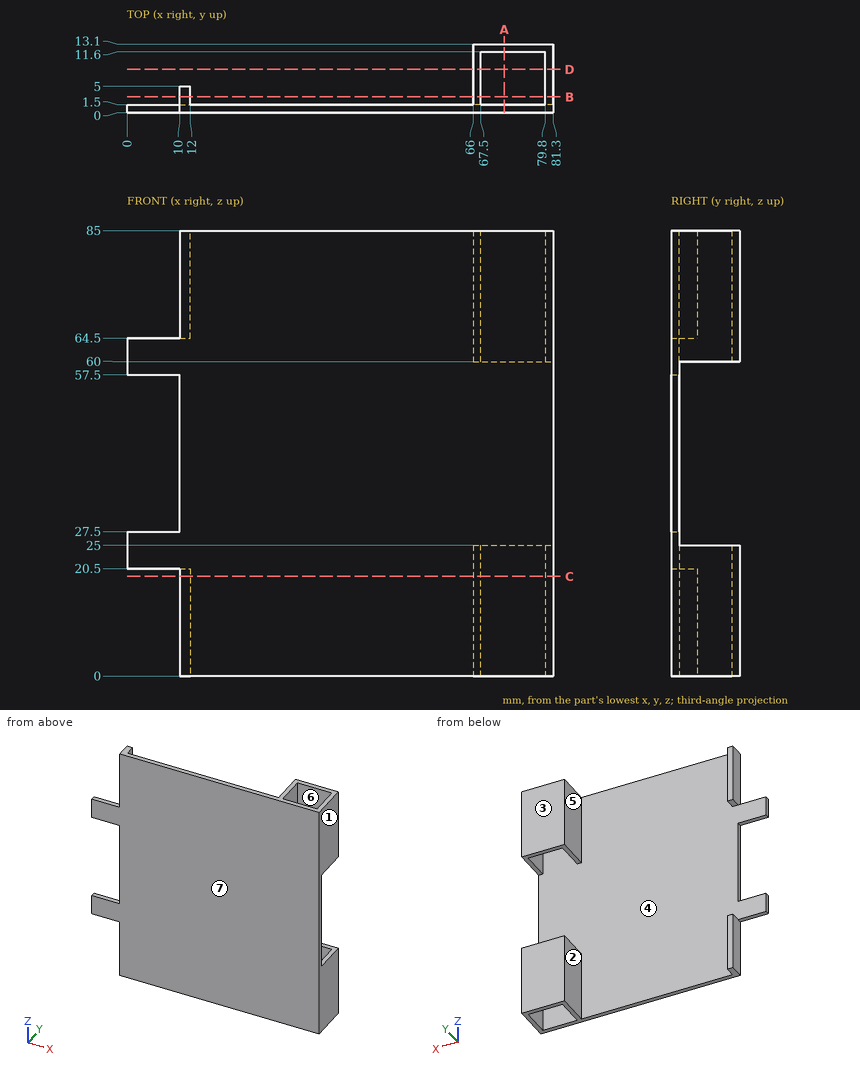
Could you check a few things on this drawing? It's one solid part, dimensions in mm from its lowest x, y, z. A direction names the side the tool comes from. Coordinates: 2 decimals unless noted, no trailing zeros. Write each loop counter-clockwise with the first axis right and the second up, starting at its lowest first coordinate (ties: lowest second). Pieces come first, ordered by that corner, then holes. Notation, with made-up numbers: M 75.25,21.25 L 83.25,21.25 A11 cw 83.25,32.25 Z; hole C -33,-27.5 d2. An arc over 180 degrees is marked long. Answer as CSV lines item,"result". Start each with the question number.
Q1. Suppose I cut it at B-B, the plane y = 3. List the corners of the cut face in (x, z) for me.
Q2. Suppose I cut it at C-C, the plane z = 19. List the corners of the cut face in (x, y) for me.
Q3. Suppose I cut it at D-D, the plane y = 8.25. List the corners of the cut face in (x, z) for me.
Q4. Will these pins go through, and if not, where does the flat tip stop? pin 1 Ø5 at (y, z) = (8.5, 18) entering from -X; pin 2 Ø4 at (y, z) = (3, 12.5) entering from -X; pin 3 Ø10 at (x, z) = (55.5, 38) entering from +Y.
Q5. I need wall thicknesses on probe 1 along X at (y, z) = (4, 80); probe 2 along X at (y, z) = (2.5, 21); probe 3 along Y at (x, z) = (31.5, 38). Which ranges of each line are inside material? Lowest first, please. Write a range as [from, to].
Q6. Suppose I cut it at A-A, the plane x = 72. List the corners of the cut face in (y, z) for me.
Q7. For the marked faces 5, 6 and 7, which set-ups out of +Z, -Z, +X, -X, +Y, -Y let a thin tool reach every point of the face, with its end or its side?
Q8. If we mould it in two halves opening along X, with no side actions, what happens to the marked faces 1, 2, 3 and 4? For each: pulls with the +X half, pulls with the -X half, needs draft (parallel to the pull), parting line crosses it, or undercut.
Entries:
1,outline,"M 10,0 L 12,0 L 12,20.5 L 10,20.5 Z; M 10,64.5 L 12,64.5 L 12,85 L 10,85 Z; M 66,0 L 67.5,0 L 67.5,25 L 66,25 Z; M 66,60 L 67.5,60 L 67.5,85 L 66,85 Z; M 79.8,0 L 81.3,0 L 81.3,25 L 79.8,25 Z; M 79.8,60 L 81.3,60 L 81.3,85 L 79.8,85 Z"
2,outline,"M 10,0 L 81.3,0 L 81.3,13.1 L 66,13.1 L 66,1.5 L 12,1.5 L 12,5 L 10,5 Z; hole M 67.5,1.5 L 79.8,1.5 L 79.8,11.6 L 67.5,11.6 Z"
3,outline,"M 66,0 L 67.5,0 L 67.5,25 L 66,25 Z; M 66,60 L 67.5,60 L 67.5,85 L 66,85 Z; M 79.8,0 L 81.3,0 L 81.3,25 L 79.8,25 Z; M 79.8,60 L 81.3,60 L 81.3,85 L 79.8,85 Z"
4,pin 1,"stops at x = 66"
4,pin 2,"stops at x = 10"
4,pin 3,"stops at y = 1.5"
5,probe 1,"x = [10, 12], [66, 67.5], [79.8, 81.3]"
5,probe 2,"x = [66, 67.5], [79.8, 81.3]"
5,probe 3,"y = [0, 1.5]"
6,outline,"M 0,0 L 1.5,0 L 1.5,85 L 0,85 Z; M 11.6,0 L 13.1,0 L 13.1,25 L 11.6,25 Z; M 11.6,60 L 13.1,60 L 13.1,85 L 11.6,85 Z"
7,face 5,"+Z, -Z, +Y"
7,face 6,"+Z, -Z"
7,face 7,"+Z, -Z, +X, -X, -Y"
8,face 1,"pulls with the +X half"
8,face 2,"undercut"
8,face 3,"needs draft"
8,face 4,"undercut"
